Can you work these out from the model? Positions are in its coordinate system, mm. Face numbers are marked on the shaded views. A direction names the side the tool comes from. Coordinates: 2 decimals unless noted, no trailing zeros. Write each loop counter-clockwise with the first axis right and the second up, starting at its lowest first coordinate (ties: lowest second). Pieces come first, ordered by that corner, then holes. Notation, with made-up numbers: (-23, -9.5) - (10, -9.5) arc R17 cw to (10, 12.5) - close; hole circle Ø7 at (-17, 59). An arc over 180 degrees is marked (long way). Write each question's results on one line, items separated by ' | '. Start each with the question number.
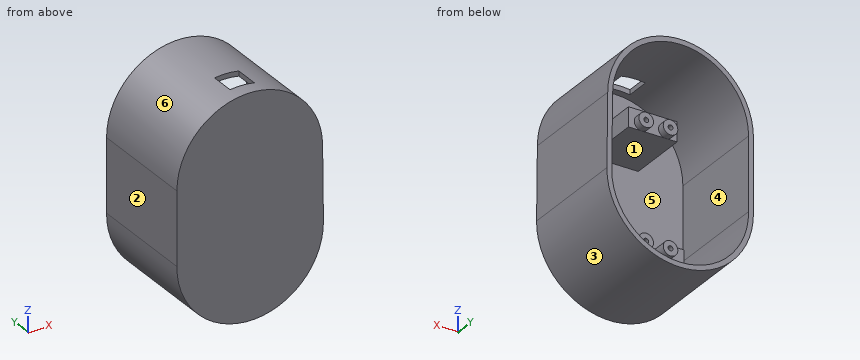
Autodesk Inventor part; units mm, degrees
ref_plane "YZ Plane" through (0, 0, 0) normal (1, 0, 0) x (0, 1, 0)
ref_plane "XZ Plane" through (0, 0, 0) normal (0, 1, 0) x (-1, 0, 0)
ref_plane "XY Plane" through (0, 0, 0) normal (0, 0, 1) x (1, 0, 0)
sketch "Sketch10" plane through (0, 0, 0) normal (0, 1, 0) x (-1, 0, 0)
  arc A0 (30, 0) -> (-30, 0) centre (0, 0) ccw
  line L0 (30, 0) -> (30, -30)
  line L1 (-30, 0) -> (-30.34, -29.9981)
  arc A1 (-30.34, -29.9981) -> (30, -30) centre (-0.17, -30.34) ccw
  point P0 (0, 30)
  point P1 (0, 30)
  dimension "d39" = 60
  dimension "d40" = 30
extrude "Extrusion10" add sketch "Sketch10" along normal blind 3
sketch "Sketch11" plane through (0, 3, 0) normal (0, 1, 0) x (1, 0, 0)
  arc A0 (-30, 0) -> (30, 0) centre (0, 0) ccw
  line L0 (-30, 30) -> (-30, 0)
  line L1 (30, 0) -> (30.34, 29.9981)
  arc A1 (30.34, 29.9981) -> (-30, 30) centre (0.17, 30.34) ccw
  line L2 (-30, 30) -> (-30, 0)
  arc A2 (-30, 0) -> (30, 0) centre (0, 0) ccw
  line L3 (-28, 30) -> (-28, 0)
  arc A3 (-28, 0) -> (28, 0) centre (0, 0) ccw
  arc A4 (28.3401, 30.0207) -> (-28, 30.0115) centre (0.17, 30.34) ccw
  line L4 (28.3401, 30.0207) -> (28, 0.0111)
  arc A5 (-28, 0) -> (28, 0.0111) centre (0, 0) ccw
  line L5 (-28, 0) -> (-28, 30.0115)
  point P0 (30, 0)
  point P1 (28, 0)
  dimension "d43" = 2
  dimension "d44" = 2
extrude "Extrusion11" add sketch "Sketch11" along normal blind 42.3
sketch "Sketch12" plane through (0, 3, 0) normal (0, 1, 0) x (1, 0, 0)
  line L0 (-5, -3.2387) -> (5, -3.2387)
  line L1 (5, -3.2387) -> (5, 44.7613)
  line L2 (5, 44.7613) -> (-5, 44.7613)
  line L3 (-5, 44.7613) -> (-5, -3.2387)
  line L4 (-5, -3.2387) -> (5, 44.7613) construction
  line L5 (5, -3.2387) -> (-5, 44.7613) construction
  circle A0 centre (-5, -3.2387) radius 3
  circle A1 centre (-5, 44.7613) radius 3
  circle A2 centre (5, 44.7613) radius 3
  circle A3 centre (5, -3.2387) radius 3
  point P0 (0, 0)
  point P1 (0, 20.7613)
  dimension "d47" = 10
  dimension "d48" = 48
  dimension "d49" = 6
  dimension "d50" = 6
  dimension "d51" = 6
  dimension "d52" = 6
extrude "Extrusion12" add sketch "Sketch12" along normal blind 28 contours L3 A0 L0 | L0 A0 L3 | A3 L1 L0 | L0 L1 A3 | A1 L2 L3 | L3 L2 A1 | A2 L2 L1 | L1 L2 A2
sketch "Sketch13" plane through (-5, 31, 3.2387) normal (0, 1, 0) x (1, 0, 0)
  circle A0 centre (0, 0) radius 3
  circle A1 centre (10, 0) radius 3
  circle A2 centre (0, 48) radius 3
  circle A3 centre (10, 48) radius 3
  circle A4 centre (0, 0) radius 1
  circle A5 centre (10, 0) radius 1
  circle A6 centre (0, 48) radius 1
  circle A7 centre (10, 48) radius 1
  point P0 (5, 3.2387)
  dimension "d55" = 2
  dimension "d56" = 2
  dimension "d57" = 2
  dimension "d58" = 2
extrude "Extrusion13" cut sketch "Sketch13" against normal blind 14 contours A4 | A5 | A6 | A7
sketch "Sketch14" plane through (0, 3, 0) normal (0, 1, 0) x (1, 0, 0)
  line L0 (-9.6197, -0.2387) -> (10.3803, -0.2387)
  circle A0 centre (5, -3.2387) radius 3
  circle A1 centre (-5, -3.2387) radius 3
  line L1 (-9.6197, -0.2387) -> (-9.6197, -8.2414)
  line L2 (-9.6197, -8.2414) -> (10.3803, -8.2414)
  line L3 (10.3803, -8.2414) -> (10.3803, -0.2387)
  circle A2 centre (-5, 44.7613) radius 3
  line L4 (-5, 47.7613) -> (-12.4823, 47.7613)
  line L5 (-12.4823, 47.7613) -> (-12.4823, 41.7613)
  line L6 (-12.4823, 41.7613) -> (-5, 41.7613)
  line L7 (0, 27.9217) -> (0, 57.8155) construction
  line L8 (5, 47.7613) -> (12.4823, 47.7613)
  line L9 (12.4823, 47.7613) -> (12.4823, 41.7613)
  line L10 (12.4823, 41.7613) -> (5, 41.7613)
  arc A3 (5, 41.7613) -> (5, 47.7613) centre (5, 44.7613) ccw
  point P0 (0, 0)
  point P1 (5, -0.2387)
  point P2 (-5, -0.2387)
  point P3 (5, 44.7613)
  dimension "d61" = 20
extrude "Extrusion14" add sketch "Sketch14" along normal blind 25 contours L0 L3 L2 L1
extrude "Extrusion15" add sketch "Sketch14" along normal blind 25 contours A2 L6 L5 L4 | L8 L9 L10 A3
sketch "Sketch15" plane through (0, 3, 0) normal (0, 1, 0) x (1, 0, 0)
  line L0 (-12.4823, 47.7613) -> (-5, 47.7613)
  line L1 (-12.4823, 47.7613) -> (-5, 47.7613)
  line L2 (-5, 47.7613) -> (-5, 50.6795)
  line L3 (-5, 50.6795) -> (-12.4823, 50.6795)
  line L4 (-12.4823, 50.6795) -> (-12.4823, 47.7613)
  point P0 (0, 0)
extrude "Extrusion16" add sketch "Sketch15" along normal blind 3
mirror "Mirror2" about plane through (0, 0, 0) normal (1, 0, 0) of "Extrusion16"
sketch "Sketch16" plane through (0, 3, 0) normal (0, 1, 0) x (1, 0, 0)
  line L0 (10.3803, -8.2414) -> (-9.6197, -8.2414)
  line L1 (-9.6197, -8.2414) -> (10.3803, -8.2414)
  line L2 (10.3803, -8.2414) -> (10.3803, -10.45)
  line L3 (10.3803, -10.45) -> (-9.6197, -10.45)
  line L4 (-9.6197, -10.45) -> (-9.6197, -8.2414)
  point P0 (0, 0)
extrude "Extrusion17" add sketch "Sketch16" along normal blind 3
sketch "Sketch17" plane through (-9.6197, 28, 8.2414) normal (0, 0, 1) x (1, 0, 0)
  line L0 (0, -22) -> (20, -22)
  line L1 (5.3464, -22) -> (15.3464, -22)
  line L2 (15.3464, -22) -> (15.3464, -12)
  line L3 (15.3464, -12) -> (5.3464, -12)
  line L4 (5.3464, -12) -> (5.3464, -22)
  point P0 (9.6197, -28)
  dimension "d70" = 10
  dimension "d71" = 10
extrude "Extrusion18" cut sketch "Sketch17" along normal blind 34.75
properties part number "Base_3DPrint"
Q1. If we section it at B-B (z = -14.5): Please give me the cut outline in (x, y), then the cut area to 3 significant figures.
Q2. If we section it at A-A (x = 0): Please give me the cut outline in (y, z).
Q3. I need wall thicknesses on line 1 along Z through (x, y) = (-5, 22.5); line 2 along X through (y, z) = (8.5, -29.5); line 3 along X through (y, z) = (25.5, 7.5). Which ranges of each line are inside material? Lowest first, please. Write a range as from..to.
Q4. I'm going to push flat-ended pins straight in: pin 1 Ø2 at (x, y) = (7, 14.5) entering from -Z; pin 2 Ø0.9 at (y, z) = (5, -49) entering from +X; pin 3 Ø1.5 at (y, z) = (21, -45.5) entering from +X. Where does each tip first touch, or does it pass through?
Q5. Thinking about a two-plate mould opening in X: for the marked faces 1, 2, 3 and 4, which applies, pulls with the +X half, pulls with the -X half, needs draft (parallel to the pull), parting line crosses it, or undercut?
Q6. For the marked faces 5 and 6, which set-ups out of +Z, -Z, +X, -X, +Y, -Y let a thin tool reach every point of the face, with its end or its side?
Q7. If we section it at C-C (x = 19): Please give me the cut outline in (y, z).
Answer list:
1) outline: (-30, 0) - (30.16, 0) - (30.16, 45.3) - (28.16, 45.3) - (28.16, 3) - (-28, 3) - (-28, 45.3) - (-30, 45.3) - close | area: 350 mm2
2) outline: (0, -60.51) - (45.3, -60.51) - (45.3, -58.51) - (3, -58.51) - (3, 0.24) - (28, 0.24) - (28, 8.24) - (6, 8.24) - (6, 10.45) - (3, 10.45) - (3, 28) - (6, 28) - (6, 30) - (0, 30) - close; (16, 28) - (45.3, 28) - (45.3, 30) - (16, 30) - close
3) line 1: z = -60.07..-58.03, -47.76..-45.76, -43.76..-41.76, 0.24..2.24, 4.24..8.24, 27.55..29.58 | line 2: x = -30..-28, 28.33..30.33 | line 3: x = -29.05..-26.98, -9.62..10.38, 26.98..29.05
4) pin 1: stops at z = -59.94 | pin 2: stops at x = 24.23 | pin 3: stops at x = 26.68
5) face 1: undercut | face 2: pulls with the -X half | face 3: parting line crosses it | face 4: undercut
6) face 5: +Y | face 6: +Z, +Y, -Y
7) outline: (0, -53.91) - (45.3, -53.91) - (45.3, -51.29) - (3, -51.29) - (3, 20.57) - (45.3, 20.57) - (45.3, 23.22) - (0, 23.22) - close
